Build history of the part. All positions in model axes, mm. Face numbers are marked on the shaded views. A direction names the side the tool comes from. Round coordinates to 2 decimals unless told otherwise and drop trailing zeros. Loops run counter-clockwise (first coordinate to the right, second up) from the corner with the lowest first, then second, coordinate; pieces in that order, holes last. Notation, with made-up numbers: (-9.75, -4) - (1.25, -4) arc R19 ccw to (1.25, 8) - close; hole circle Ø10 at (-24.5, -15.5). An arc over 180 degrees is marked (long way). Put each result on its own line as item: value. Start each with the question number.
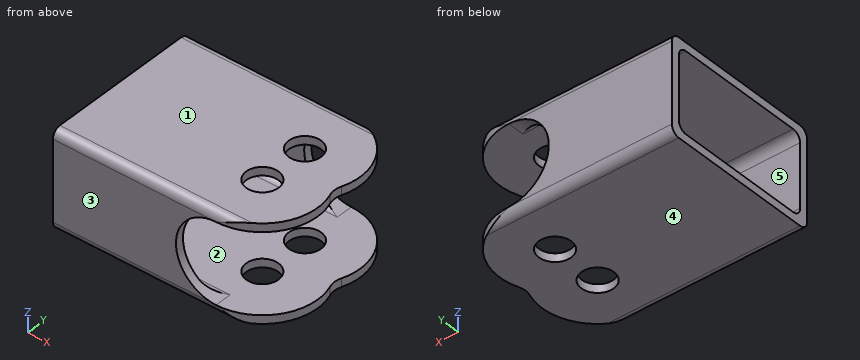
from build123d import *

# Parameters (mm, degrees)
SQUARE_TUBE_1_5X0_75_0_065_4130_TUBE_1_DEPTH = 43.474215441
SKETCH3_R                                    = 3.175
CUT_EXTRUDE1_DEPTH                           = 51.049231095
CUT_EXTRUDE2_DEPTH                           = 55.229578607
FILLET1_R                                    = 3.81


with BuildPart() as part:
    # Sketch2 → Square tube 1.5X0.75-0.065 4130 TUBE(1) (new body)
    with BuildSketch(Plane.YZ):
        with BuildLine():
            Line((-14.224, -9.525), (14.224, -9.525))
            ThreePointArc((14.224, -9.525), (15.391433296, -9.041433296), (15.875, -7.874))
            Line((15.875, -7.874), (15.875, 7.874))
            ThreePointArc((15.875, 7.874), (15.391433296, 9.041433296), (14.224, 9.525))
            Line((14.224, 9.525), (-14.224, 9.525))
            ThreePointArc((-14.224, 9.525), (-15.391433296, 9.041433296), (-15.875, 7.874))
            Line((-15.875, 7.874), (-15.875, -7.874))
            ThreePointArc((-15.875, -7.874), (-15.391433296, -9.041433296), (-14.224, -9.525))
        make_face()
        with BuildLine():
            Line((-12.573, 7.874), (12.573, 7.874))
            ThreePointArc((12.573, 7.874), (13.740433296, 7.390433296), (14.224, 6.223))
            Line((14.224, 6.223), (14.224, -6.223))
            ThreePointArc((14.224, -6.223), (13.740433296, -7.390433296), (12.573, -7.874))
            Line((12.573, -7.874), (-12.573, -7.874))
            ThreePointArc((-12.573, -7.874), (-13.740433296, -7.390433296), (-14.224, -6.223))
            Line((-14.224, -6.223), (-14.224, 6.223))
            ThreePointArc((-14.224, 6.223), (-13.740433296, 7.390433296), (-12.573, 7.874))
        make_face(mode=Mode.SUBTRACT)
    extrude(amount=SQUARE_TUBE_1_5X0_75_0_065_4130_TUBE_1_DEPTH)

    # Sketch3 → Cut-Extrude1 (cut, through all)
    with BuildSketch(Plane.XY.offset(9.525)):
        with Locations((32.044215441, 5)):
            Circle(SKETCH3_R)
        with Locations((32.044215441, -5)):
            Circle(SKETCH3_R)
        with BuildLine():
            Line((43.474215441, -15.875), (32.044215441, -15.875))
            ThreePointArc((32.044215441, -15.875), (41.335087978, -10.652018445), (41.701628397, 0))
            ThreePointArc((41.701628397, 0), (41.335087978, 10.652018445), (32.044215441, 15.875))
            Line((32.044215441, 15.875), (43.474215441, 15.875))
            Line((43.474215441, 15.875), (43.474215441, -15.875))
        make_face()
    extrude(amount=-CUT_EXTRUDE1_DEPTH, mode=Mode.SUBTRACT)

    # Sketch4 → Cut-Extrude2 (cut, through all)
    with BuildSketch(Plane(origin=(0, 15.875, 0), x_dir=(1, 0, 0), z_dir=(0, 1, 0))):
        with BuildLine():
            Line((39.849040615, -7.874), (32.044215441, -7.874))
            ThreePointArc((32.044215441, -7.874), (24.170215441, 0), (32.044215441, 7.874))
            Line((32.044215441, 7.874), (39.849040615, 7.874))
            Line((39.849040615, 7.874), (39.849040615, -7.874))
        make_face()
    extrude(amount=-CUT_EXTRUDE2_DEPTH, mode=Mode.SUBTRACT)

    # Fillet1
    fillet1_edges = [part.edges().sort_by_distance(p)[0] for p in [
        (41.701628397, 0, -8.6995),
        (41.701628397, 0, 8.6995),
    ]]
    fillet(fillet1_edges, radius=FILLET1_R)


solid = part.part
Item 1: Slice it at A-A (y = -5). Give the cut face in (x, z) (3 decimals), plus the area to 3 significant figures.
Item 2: Which spindle directions (+Z, -Z, +X, -X, +Y, -Y) get a long thin tool onto all of the face, cutting with end or side? Do the marked faces 4 and 5. Say none if no direction does.
Item 3: Slice it at C-C (x = 22). Give the cut face in (y, z) (3 decimals).
Item 4: Slice it at D-D (x = 34.5). Give the cut face in (y, z) (3 decimals).
Item 5: Drill centre lines: probe 1 along Z at (x, y) = (11, -5) (3 decimals); probe 2 along Y at (x, z) = (11, -2.5) (3 decimals); probe 3 along Y at (x, z) = (31, 8). Where is each one in solid material? Low to high. Write a range as [from, to].
Item 6: Slice it at B-B (z = 0). Give the cut face in (x, y) (3 decimals).
Item 7: Two-plate mould, pull along Y, no slides. Class the marked faces 1, 2 and 3: pulls with the +Y half, pulls with the -Y half, needs draft (parallel to the pull), parting line crosses it, or undercut.
Computed values:
1. outline: (0, -9.525) - (28.869, -9.525) - (28.869, -7.874) - (0, -7.874) - close; (0, 7.874) - (28.869, 7.874) - (28.869, 9.525) - (0, 9.525) - close; (35.219, -9.525) - (42.919, -9.525) - (42.919, -7.874) - (35.219, -7.874) - close; (35.219, 7.874) - (42.919, 7.874) - (42.919, 9.525) - (35.219, 9.525) - close
1. area: 121 mm^2
2. face 4: -Z, +X, -X, +Y, -Y
2. face 5: +X, -X
3. outline: (-15.875, -7.874) arc R1.651 ccw to (-14.224, -9.525) - (14.224, -9.525) arc R1.651 ccw to (15.875, -7.874) - (15.875, 7.874) arc R1.651 ccw to (14.224, 9.525) - (-14.224, 9.525) arc R1.651 ccw to (-15.875, 7.874) - close; hole (-14.224, -6.223) arc R1.651 ccw to (-12.573, -7.874) - (12.573, -7.874) arc R1.651 ccw to (14.224, -6.223) - (14.224, 6.223) arc R1.651 ccw to (12.573, 7.874) - (-12.573, 7.874) arc R1.651 ccw to (-14.224, 6.223) - close
4. outline: (-15.594, -8.795) arc R1.651 ccw to (-14.224, -9.525) - (-7.012, -9.525) - (-7.012, -7.874) - (-15.594, -7.874) - close; (-15.594, 7.874) - (-7.012, 7.874) - (-7.012, 9.525) - (-14.224, 9.525) arc R1.651 ccw to (-15.594, 8.795) - close; (-2.988, -9.525) - (2.988, -9.525) - (2.988, -7.874) - (-2.988, -7.874) - close; (-2.988, 7.874) - (2.988, 7.874) - (2.988, 9.525) - (-2.988, 9.525) - close; (7.012, -9.525) - (14.224, -9.525) arc R1.651 ccw to (15.594, -8.795) - (15.594, -7.874) - (7.012, -7.874) - close; (7.012, 7.874) - (15.594, 7.874) - (15.594, 8.795) arc R1.651 ccw to (14.224, 9.525) - (7.012, 9.525) - close
5. probe 1: z = [-9.525, -7.874], [7.874, 9.525]
5. probe 2: y = [-15.875, -14.224], [14.224, 15.875]
5. probe 3: y = [-15.87, -8], [-2, 2], [8, 15.87]
6. outline: (0, -15.875) - (24.17, -15.875) - (24.17, -14.224) - (0, -14.224) - close; (0, 14.224) - (24.17, 14.224) - (24.17, 15.875) - (0, 15.875) - close
7. face 1: needs draft
7. face 2: undercut
7. face 3: pulls with the -Y half
